```python
from build123d import *

# Parameters (mm, degrees)
SKETCH1_R           = 57.000000046
SKETCH1_R_2         = 45.72
BOSS_EXTRUDE1_DEPTH = 15
SKETCH3_R           = 49.001810824
SKETCH3_R_2         = 37.55
BOSS_EXTRUDE3_DEPTH = 15
CUT_EXTRUDE1_REACH  = 83.994
SKETCH4_R           = 2
SKETCH6_R           = 1.5
CUT_EXTRUDE2_DEPTH  = 82.993902276
CIRPATTERN2_COUNT   = 8
CIRPATTERN1_COUNT   = 12
SKETCH10_R          = 57.000000046
SKETCH10_R_2        = 42.000000046
SKETCH10_R_3        = 1.5
SKETCH10_R_4        = 2
BOSS_EXTRUDE4_DEPTH = 7
SKETCH12_R          = 2.35
CUT_EXTRUDE3_DEPTH  = 6.5
SKETCH13_R          = 2.925
CUT_EXTRUDE4_DEPTH  = 2
SKETCH14_R          = 2.85
CUT_EXTRUDE5_DEPTH  = 9


with BuildPart() as part:
    # Sketch1 → Boss-Extrude1 (new body)
    with BuildSketch(Plane(origin=(0, 0, 0), x_dir=(0, 0, -1), z_dir=(1, 0, 0))):
        Circle(SKETCH1_R)
        Circle(SKETCH1_R_2, mode=Mode.SUBTRACT)
    extrude(amount=BOSS_EXTRUDE1_DEPTH)

    # Sketch3 → Boss-Extrude3 (add)
    with BuildSketch(Plane.ZY):
        Circle(SKETCH3_R)
        Circle(SKETCH3_R_2, mode=Mode.SUBTRACT)
    extrude(amount=-BOSS_EXTRUDE3_DEPTH)

    # Sketch4 → Cut-Extrude1 (cut, up to next)
    with BuildSketch(Plane(origin=(15, 0, 0), x_dir=(0, 0, -1), z_dir=(1, 0, 0)), mode=Mode.PRIVATE) as cut_extrude1_sk1:
        with Locations((0, 50)):
            Circle(SKETCH4_R)
    cut_extrude1_tool1 = extrude(cut_extrude1_sk1.sketch, amount=-CUT_EXTRUDE1_REACH, mode=Mode.PRIVATE) & part.part
    cut_extrude1 = cut_extrude1_tool1.solids().sort_by_distance((15, 50, 0))[0]
    add(cut_extrude1, mode=Mode.SUBTRACT)

    # Sketch6 → Cut-Extrude2 (cut, through all)
    with BuildSketch(Plane(origin=(15, 0, 0), x_dir=(0, 0, -1), z_dir=(1, 0, 0))):
        with Locations((-5.891755706, 44.108244294)):
            Circle(SKETCH6_R)
    cut_extrude2 = extrude(amount=-CUT_EXTRUDE2_DEPTH, mode=Mode.SUBTRACT)

    # CirPattern2: Cut-Extrude2 ×8 about axis
    cirpattern2_axis = Axis((0, 0, 0), (1, 0, 0))
    for i in range(1, CIRPATTERN2_COUNT):
        add(cut_extrude2.rotate(cirpattern2_axis, i * 360 / CIRPATTERN2_COUNT), mode=Mode.SUBTRACT)

    # CirPattern1: Cut-Extrude1 ×12 about axis
    cirpattern1_axis = Axis((0, 0, 0), (1, 0, 0))
    for i in range(1, CIRPATTERN1_COUNT):
        add(cut_extrude1.rotate(cirpattern1_axis, i * 360 / CIRPATTERN1_COUNT), mode=Mode.SUBTRACT)

    # Sketch10 → Boss-Extrude4 (add)
    with BuildSketch(Plane.ZY):
        Circle(SKETCH10_R)
        Circle(SKETCH10_R_2, mode=Mode.SUBTRACT)
        with Locations(Location((-27.023138234, 35.355339059, 0), (0, 0, 225))):
            Circle(SKETCH10_R_3, mode=Mode.SUBTRACT)
        with Locations(Location((5.891755706, 44.108244294, 0), (0, 0, 180))):
            Circle(SKETCH10_R_3, mode=Mode.SUBTRACT)
        with Locations(Location((35.355339059, 27.023138234, 0), (0, 0, 135))):
            Circle(SKETCH10_R_3, mode=Mode.SUBTRACT)
        with Locations(Location((44.108244294, -5.891755706, 0), (0, 0, 90))):
            Circle(SKETCH10_R_3, mode=Mode.SUBTRACT)
        with Locations(Location((27.023138234, -35.355339059, 0), (0, 0, 45))):
            Circle(SKETCH10_R_3, mode=Mode.SUBTRACT)
        with Locations(Location((-44.108244294, 5.891755706, 0), (0, 0, 270))):
            Circle(SKETCH10_R_3, mode=Mode.SUBTRACT)
        with Locations(Location((-35.355339059, -27.023138234, 0), (0, 0, 315))):
            Circle(SKETCH10_R_3, mode=Mode.SUBTRACT)
        with Locations((-5.891755706, -44.108244294)):
            Circle(SKETCH10_R_3, mode=Mode.SUBTRACT)
        with Locations(Location((-25, 43.301270189, 0), (0, 0, 180))):
            Circle(SKETCH10_R_4, mode=Mode.SUBTRACT)
        with Locations(Location((0, 50, 0), (0, 0, 180))):
            Circle(SKETCH10_R_4, mode=Mode.SUBTRACT)
        with Locations(Location((25, 43.301270189, 0), (0, 0, 180))):
            Circle(SKETCH10_R_4, mode=Mode.SUBTRACT)
        with Locations(Location((43.301270189, 25, 0), (0, 0, 180))):
            Circle(SKETCH10_R_4, mode=Mode.SUBTRACT)
        with Locations(Location((50, 0, 0), (0, 0, 180))):
            Circle(SKETCH10_R_4, mode=Mode.SUBTRACT)
        with Locations(Location((43.301270189, -25, 0), (0, 0, 180))):
            Circle(SKETCH10_R_4, mode=Mode.SUBTRACT)
        with Locations(Location((25, -43.301270189, 0), (0, 0, 180))):
            Circle(SKETCH10_R_4, mode=Mode.SUBTRACT)
        with Locations(Location((0, -50, 0), (0, 0, 180))):
            Circle(SKETCH10_R_4, mode=Mode.SUBTRACT)
        with Locations(Location((-25, -43.301270189, 0), (0, 0, 180))):
            Circle(SKETCH10_R_4, mode=Mode.SUBTRACT)
        with Locations(Location((-43.301270189, -25, 0), (0, 0, 180))):
            Circle(SKETCH10_R_4, mode=Mode.SUBTRACT)
        with Locations(Location((-50, 0, 0), (0, 0, 180))):
            Circle(SKETCH10_R_4, mode=Mode.SUBTRACT)
        with Locations(Location((-43.301270189, 25, 0), (0, 0, 180))):
            Circle(SKETCH10_R_4, mode=Mode.SUBTRACT)
    extrude(amount=BOSS_EXTRUDE4_DEPTH)

    # Sketch12 → Cut-Extrude3 (cut)
    with BuildSketch(Plane(origin=(15, 0, 0), x_dir=(0, 0, -1), z_dir=(1, 0, 0))):
        with Locations((-35.355339059, 27.023138234)):
            Circle(SKETCH12_R)
        with Locations((-5.891755706, 44.108244294)):
            Circle(SKETCH12_R)
        with Locations((27.023138234, 35.355339059)):
            Circle(SKETCH12_R)
        with Locations((44.108244294, 5.891755706)):
            Circle(SKETCH12_R)
        with Locations((35.355339059, -27.023138234)):
            Circle(SKETCH12_R)
        with Locations((5.891755706, -44.108244294)):
            Circle(SKETCH12_R)
        with Locations((-27.023138234, -35.355339059)):
            Circle(SKETCH12_R)
        with Locations((-44.108244294, -5.891755706)):
            Circle(SKETCH12_R)
    extrude(amount=-CUT_EXTRUDE3_DEPTH, mode=Mode.SUBTRACT)

    # Sketch13 → Cut-Extrude4 (cut)
    with BuildSketch(Plane(origin=(15, 0, 0), x_dir=(0, 0, -1), z_dir=(1, 0, 0))):
        with Locations((-35.355339059, 27.023138234)):
            Circle(SKETCH13_R)
        with Locations((-5.891755706, 44.108244294)):
            Circle(SKETCH13_R)
        with Locations((27.023138234, 35.355339059)):
            Circle(SKETCH13_R)
        with Locations((44.108244294, 5.891755706)):
            Circle(SKETCH13_R)
        with Locations((35.355339059, -27.023138234)):
            Circle(SKETCH13_R)
        with Locations((5.891755706, -44.108244294)):
            Circle(SKETCH13_R)
        with Locations((-27.023138234, -35.355339059)):
            Circle(SKETCH13_R)
        with Locations((-44.108244294, -5.891755706)):
            Circle(SKETCH13_R)
    extrude(amount=-CUT_EXTRUDE4_DEPTH, mode=Mode.SUBTRACT)

    # Sketch14 → Cut-Extrude5 (cut)
    with BuildSketch(Plane(origin=(15, 0, 0), x_dir=(0, 0, -1), z_dir=(1, 0, 0))):
        with Locations((-43.301270189, 25)):
            Circle(SKETCH14_R)
        with Locations((-25, 43.301270189)):
            Circle(SKETCH14_R)
        with Locations((0, 50)):
            Circle(SKETCH14_R)
        with Locations((25, 43.301270189)):
            Circle(SKETCH14_R)
        with Locations((43.301270189, 25)):
            Circle(SKETCH14_R)
        with Locations((50, 0)):
            Circle(SKETCH14_R)
        with Locations((43.301270189, -25)):
            Circle(SKETCH14_R)
        with Locations((25, -43.301270189)):
            Circle(SKETCH14_R)
        with Locations((0, -50)):
            Circle(SKETCH14_R)
        with Locations((-25, -43.301270189)):
            Circle(SKETCH14_R)
        with Locations((-43.301270189, -25)):
            Circle(SKETCH14_R)
        with Locations((-50, 0)):
            Circle(SKETCH14_R)
    extrude(amount=-CUT_EXTRUDE5_DEPTH, mode=Mode.SUBTRACT)


solid = part.part
```
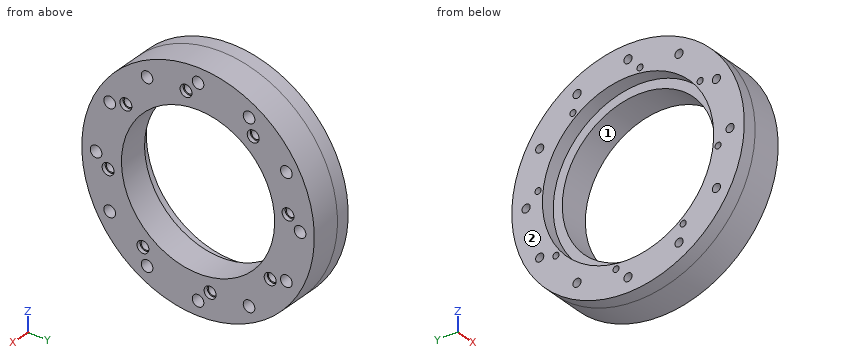
Geometry check sheet. Reference: the model listing, model coordinates, mm. Face numbers are marked on the shaded views. Coordinates: 2 decimals unless noted, no trailing zeros. Order: outer loops, then holes, each group sorted by start corner. A loop starts at its lowest first (then second) coordinate and runs counter-clockwise, first axis right, second up.
Item 1: Mould release check, pull along Y, two halves, no side actions. Record for the marked faces 1 and 2: released by +Y, released by -Y, zero draft, split by the parting line, or undercut.
Item 2: Scan lines: line 1 along Y through (x, z) = (7.75, 2.5); line 2 along Y through (x, z) = (1.5, 28); line 3 along Y through (x, z) = (8.75, -5.5). Record each from-to range of solid material in increasing order.
Item 3: Section check C-C (y = -50). Enter the section's corners in (x, z).
Item 4: Section check A-A (z = 0). Enter the section's corners in (x, y).
Item 5: Section check B-B (x = -4.5). Count the separate pieces of the cut face and the enclosed holes in it, plus the area to 3 significant figures.
Item 6: Depth check by flat-ended pin: pin 1 (8 mm diameter, centred on x = 0, z = 9, fed in from +Y); pin 2 (12 mm diameter, centred on x = 10, y = -43, fed in from +Z); pin 3 (2 mm diameter, centred on x = 12.5, y = -30.5, fed in from +Z). Enter the tip coordinate at first touch or a pass-through.
Check sheet entries:
1. face 1: undercut
1. face 2: zero draft
2. line 1: y = -56.95 to -51.37, -48.63 to -37.47, 37.47 to 48.63, 51.37 to 56.95
2. line 2: y = -49.65 to -36.49, -34.22 to -25.02, 25.02 to 49.65
2. line 3: y = -56.73 to -46.43, -41.79 to -37.15, 37.15 to 56.73
3. outline: (-7, -27.37) - (15, -27.37) - (15, -2.85) - (6, -2.85) - (6, -2) - (-7, -2) - close; (-7, 2) - (6, 2) - (6, 2.85) - (15, 2.85) - (15, 27.37) - (-7, 27.37) - close
4. outline: (-7, -57) - (15, -57) - (15, -52.85) - (6, -52.85) - (6, -52) - (-7, -52) - close; (-7, -48) - (6, -48) - (6, -47.15) - (15, -47.15) - (15, -37.55) - (0, -37.55) - (0, -42) - (-7, -42) - close; (-7, 42) - (0, 42) - (0, 37.55) - (15, 37.55) - (15, 47.15) - (6, 47.15) - (6, 48) - (-7, 48) - close; (-7, 52) - (6, 52) - (6, 52.85) - (15, 52.85) - (15, 57) - (-7, 57) - close
5. separate pieces: 1
5. enclosed holes: 21
5. area: 4,460 mm2
6. pin 1: stops at y = 56.78
6. pin 2: stops at z = 43.36
6. pin 3: stops at z = 48.77
